Autodesk Inventor part; units mm, degrees
ref_plane "YZ Plane" through (0, 0, 0) normal (1, 0, 0) x (0, 1, 0)
ref_plane "XZ Plane" through (0, 0, 0) normal (0, 1, 0) x (-1, 0, 0)
ref_plane "XY Plane" through (0, 0, 0) normal (0, 0, 1) x (1, 0, 0)
sketch "Sketch1" plane through (0, 0, 0) normal (0, 0, 1) x (1, 0, 0)
  line L0 (-339.725, 0) -> (339.725, 0)
  line L1 (339.725, 0) -> (339.725, 47.625)
  line L2 (339.725, 47.625) -> (566.1025, 47.625)
  line L3 (601.6625, 59.2709) -> (601.6625, 131.2291)
  line L4 (566.1025, 142.875) -> (-566.1025, 142.875)
  line L5 (-601.6625, 131.2291) -> (-601.6625, 59.2709)
  line L6 (-566.1025, 47.625) -> (-339.725, 47.625)
  line L7 (-339.725, 47.625) -> (-339.725, 0)
  line L8 (566.1025, 47.625) -> (566.1025, 48.9204)
  arc A0 (571.2291, 54.3232) -> (566.1025, 48.9204) centre (571.5127, 48.9204) ccw
  line L9 (571.2291, 54.3232) -> (598.317, 55.7452)
  arc A1 (598.317, 55.7452) -> (601.6625, 59.2709) centre (598.1319, 59.2709) ccw
  line L10 (566.1025, 142.875) -> (566.1025, 141.5796)
  arc A2 (566.1025, 141.5796) -> (571.2291, 136.1768) centre (571.5127, 141.5796) ccw
  line L11 (571.2291, 136.1768) -> (598.317, 134.7548)
  arc A3 (601.6625, 131.2291) -> (598.317, 134.7548) centre (598.1319, 131.2291) ccw
  line L12 (-566.1025, 142.875) -> (-566.1025, 141.5796)
  arc A4 (-571.2291, 136.1768) -> (-566.1025, 141.5796) centre (-571.5127, 141.5796) ccw
  line L13 (-571.2291, 136.1768) -> (-598.317, 134.7548)
  arc A5 (-598.317, 134.7548) -> (-601.6625, 131.2291) centre (-598.1319, 131.2291) ccw
  line L14 (-566.1025, 47.625) -> (-566.1025, 48.9204)
  arc A6 (-566.1025, 48.9204) -> (-571.2291, 54.3232) centre (-571.5127, 48.9204) ccw
  line L15 (-571.2291, 54.3232) -> (-598.317, 55.7452)
  arc A7 (-601.6625, 59.2709) -> (-598.317, 55.7452) centre (-598.1319, 59.2709) ccw
  point P0 (0, 0)
  point P1 (0, 0)
  dimension "d0" = 679.45
  dimension "d1" = 1203.325
  dimension "d2" = 47.625
  dimension "d3" = 95.25
  dimension "d4" = 71.9582
  dimension "d8" = 3.5306
  dimension "d9" = 5.4102
  dimension "d10" = 35.56
  dimension "d11" = 1.2954
extrude "Extrusion1" add sketch "Sketch1" along normal blind 6.35
fillet "Fillet1" radius 15.875 2 edges at (-339.725, 47.625, 3.175) (339.725, 47.625, 3.175)
properties part number "A1-18002-100-40 Pocket door plate" material "Steel, Mild"
Input: part model. Units: mm. Frame: model coordinates. Give positions to 0.01 mm unless a question says otherwise; leave off trailing zeros. Write each loop counter-clockwise with the first axis right and the second up, starting at its lowest first coordinate (ties: lowest second). Pieces come first, ordered by that corner, then holes.
Q1. First-contact query: P1, Ø1, axis at y = 142, z = 2, coming from the +X side; P2, Ø2, axis at y = 31.5, z = 1.5, coming from the +X side; P3, Ø1, axis at y = 142, z = 2, coming from the -X side. Flat tips, straight axial feed; report the tip coordinate or a pass-through.
Q2. Section B-B, the plane y = 20.5. Output: boundary loops of the cut face in (x, z) (3 decimals), plus the area to 3 significant figures.
Q3. Section C-C, the plane x = -464. Output: boundary loops of the cut face in (y, z) (3 decimals).
Q4. Material intervals for probe 1 along Y at (x, z) = (-490, 6) (3 decimals); probe 2 along X at (y, z) = (25, 5.5) (3 decimals); probe 3 along X at (y, z) = (50.5, 2.75), sorted ascending.
Filled in:
1. P1: stops at x = 566.1
1. P2: stops at x = 339.74
1. P3: stops at x = -566.1
2. outline: (-339.725, 0) - (339.725, 0) - (339.725, 6.35) - (-339.725, 6.35) - close
2. area: 4,310 mm2
3. outline: (47.625, 0) - (142.875, 0) - (142.875, 6.35) - (47.625, 6.35) - close
4. probe 1: y = 47.625 to 142.875
4. probe 2: x = -339.725 to 339.725
4. probe 3: x = -566.34 to 566.34
